Verification items for the finished model (mm, model axes). Face numbers are marked on the shaded views. A direction names the side the tool comes from. Round coordinates to 2 decimals unless told otherwise and drop trailing zeros. Order: outer loops, then holes, each group sorted by start corner. A loop starts at its lowest first (then second) coordinate and runs counter-clockwise, first axis right, second up. Notation, with made-up numbers: M -22,34 L 19,34 A19 ccw 19,52 Z; hole C -9.5,25.25 d5. An arc over 180 degrees is marked long. Return JSON: item names as keys, results as strings. Group by question number.
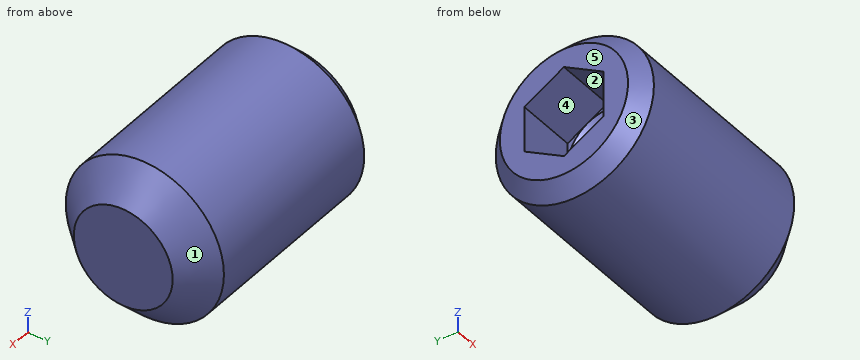
from build123d import *

# Parameters (mm, degrees)
HEXAGONSOCKET_DEPTH = 1.5


with BuildPart() as part:
    # Sketch1 → Base (revolve)
    with BuildSketch(Plane.XY):
        Polygon((0, 0), (6, 0), (6, 1.25), (5.25, 2), (0.379, 2), (0, 1.621), align=None)
    revolve(axis=Axis((-10.745014543, 0, 0), (1, 0, 0)))

    # Sketch2 → HexagonSocket (cut)
    with BuildSketch(Plane(origin=(0, -0.021932325, 0.010138848), x_dir=(0, 0, 1), z_dir=(-1, 0, 0))):
        Polygon((1.14456169, 0.021932325), (0.567211421, 1.021932325), (-0.587489117, 1.021932325), (-1.164839386, 0.021932325), (-0.587489117, -0.978067675), (0.567211421, -0.978067675), align=None)
    extrude(amount=-HEXAGONSOCKET_DEPTH, mode=Mode.SUBTRACT)

    # Sketch3 → Cut-Revolve1 (revolve, cut)
    with BuildSketch(Plane.XY):
        Polygon((1.5, 1), (2.077350269, 0), (1.5, 0), align=None)
    revolve(axis=Axis((-3.144113667, 0, 0), (1, 0, 0)), mode=Mode.SUBTRACT)


solid = part.part
1. Draft check along Y on the marked faces 3, 4 and 5. Enter one of: +Y half, -Y half, draft (parallel to the pull), parting line (faces both ways), or undercut.
2. Thickness scan on line 1 along Z through (x, y) = (0.6, 0.5); line 2 along Y through (x, z) = (5.15, 0.95); line 3 along Y through (x, z) = (3.05, 1.8). Record the ranges inside material, lowest first. Write a range as from..to.
3. Cross-section at B-B (x = 3.7). Enter the section's corners in (y, z), plus the area to 3 significant figures.
4. Access from +Z, -Z, +X, -X, +Y, -Y to the whole of each face (thin tool, end or side, straight path). Record for the marked faces 1 and 2.
5. Cross-section at C-C (x = 5.5). Enter the section's corners in (y, z).
6. Cross-section at A-A (x = 1.1). Enter the section's corners in (y, z).
Computed:
{
 "1": {"face 3": "parting line", "face 4": "undercut", "face 5": "draft"},
 "2": {"line 1": "z = -1.94..-0.87, 0.87..1.94", "line 2": "y = -1.76..1.76", "line 3": "y = -0.87..0.87"},
 "3": {"outline": "C 0,0 d4", "area": "12.6 mm²"},
 "4": {"face 1": "+X", "face 2": "-X"},
 "5": {"outline": "C 0,0 d3.5"},
 "6": {"outline": "C 0,0 d4; hole M -1,-0.58 L 0,-1.15 L 1,-0.58 L 1,0.58 L 0,1.15 L -1,0.58 Z"}
}
